Geometry check sheet. Reference: the model listing, model coordinates, mm. Face numbers are marked on the shaded views. A direction names the side the tool comes from. Coordinates: 2 decimals unless noted, no trailing zeros. Order: outer loops, then holes, each group sorted by start corner. A loop starts at its lowest first (then second) coordinate and runs counter-clockwise, first axis right, second up. Notation, with made-up numbers: (7.5, 83) - (22.5, 83) arc R25 cw to (22.5, 95) - close; hole circle Ø4 at (57.25, -14). An arc over 180 degrees is marked (long way). Use CSV: the item, a comma, the result in double quotes. Start each with the question number.
1) Thickness scan on probe 1 along X at (y, z) = (157, 1.2); probe 2 along Y at (x, z) = (15, 4.75); probe 3 along Y at (x, z) = (37.5, 3.3). Record the ranges inside material, lowest first. Write a range as [from, to].
2) Draft check along Y on the marked faces 3, 4 and 5. Enter one of: released by +Y, released by -Y, zero draft, split by the parting line, or undercut.
3) Tool access check on the marked faces 1 and 2. Record the directions out of +Z, -Z, +X, -X, +Y, -Y that give a thin tool (end or side, any length) a straight path to the whole face; none if there is none.
4) Depth check by flat-ended pin: P1, Ø3, axis at x = 2.5, y = 8.5, coming from the -Z side; P2, Ø2, axis at x = 27.5, z = 5.5, coming from the -Y side; P3, Ø0.8, axis at x = 37.5, z = 7.5, coming from the -Y side. Enter the tip coordinate at first touch or a pass-through.
5) Sectioned sample at A-A, the plane y = 55. Record the cut outline in (x, z).
from build123d import *

# Parameters (mm, degrees)
SKETCH_W        = 50
SKETCH_H        = 160
PAD_DEPTH       = 10
POCKET_DEPTH    = 7
SKETCH003_R     = 1.6
POCKET002_DEPTH = 10
POCKET003_DEPTH = 10
SKETCH005_W     = 6.1
SKETCH005_H     = 160
POCKET004_DEPTH = 3
POCKET005_DEPTH = 5.9
SKETCH007_W     = 160
SKETCH007_H     = 4.1
POCKET006_DEPTH = 5.9
SKETCH008_W     = 30
SKETCH008_H     = 140
POCKET007_DEPTH = 7
SKETCH009_W     = 5.7
SKETCH009_H     = 2.6
POCKET008_DEPTH = 6.15
SKETCH010_R     = 1.6
POCKET009_DEPTH = 10
SKETCH011_R     = 1.6
POCKET010_DEPTH = 10


with BuildPart() as part:
    # Sketch → Pad (new body)
    with BuildSketch(Plane.XY):
        with Locations((25, 80)):
            Rectangle(SKETCH_W, SKETCH_H)
    extrude(amount=PAD_DEPTH)

    # Sketch001 (on Face6 of Pad) → Pocket (cut)
    with BuildSketch(Plane.XY.offset(10)):
        Polygon((17.4, 6.1), (32.6, 6.1), (30.1, 0), (19.9, 0), align=None)
        Polygon((42.4, 6.1), (57.6, 6.1), (55.1, 0), (44.9, 0), align=None)
        Polygon((-7.6, 6.1), (7.6, 6.1), (5.1, 0), (-5.1, 0), align=None)
        Polygon((32.2, 153.9), (17.4, 153.9), (19.9, 160), (29.7, 160), align=None)
        Polygon((7.2, 153.9), (-7.6, 153.9), (-5.1, 160), (4.7, 160), align=None)
        Polygon((57.2, 153.9), (42.4, 153.9), (44.9, 160), (54.7, 160), align=None)
    extrude(amount=-POCKET_DEPTH, mode=Mode.SUBTRACT)

    # Sketch003 → Pocket002 (cut)
    with BuildSketch(Plane.XY.offset(10)):
        with Locations((12.5, 157)):
            Circle(SKETCH003_R)
        with Locations((37.5, 157)):
            Circle(SKETCH003_R)
        with Locations((12.5, 3)):
            Circle(SKETCH003_R)
        with Locations((37.5, 3)):
            Circle(SKETCH003_R)
    extrude(amount=-POCKET002_DEPTH, mode=Mode.SUBTRACT)

    # Sketch004 (on Face2 of Pocket002) → Pocket003 (cut)
    with BuildSketch(Plane(origin=(0, 0, 0), x_dir=(1, 0, 0), z_dir=(0, 0, -1))):
        Polygon((43.9, -84.9), (43.9, -100.1), (50, -97.6), (50, -87.4), align=None)
        Polygon((43.9, -59.9), (43.9, -75.1), (50, -72.6), (50, -62.4), align=None)
        Polygon((43.9, -34.9), (43.9, -50.1), (50, -47.6), (50, -37.4), align=None)
        Polygon((43.9, -9.9), (43.9, -25.1), (50, -22.6), (50, -12.4), align=None)
        Polygon((43.9, -134.9), (43.9, -150.1), (50, -147.6), (50, -137.4), align=None)
        Polygon((43.9, -109.9), (43.9, -125.1), (50, -122.6), (50, -112.4), align=None)
    extrude(amount=-POCKET003_DEPTH, mode=Mode.SUBTRACT)

    # Sketch005 (on Face2 of Pocket003) → Pocket004 (cut)
    with BuildSketch(Plane(origin=(0, 0, 0), x_dir=(1, 0, 0), z_dir=(0, 0, -1))):
        with Locations((46.95, -80)):
            Rectangle(SKETCH005_W, SKETCH005_H)
    extrude(amount=-POCKET004_DEPTH, mode=Mode.SUBTRACT)

    # Sketch006 (on Face12 of Pocket004) → Pocket005 (cut)
    with BuildSketch(Plane(origin=(0, 0, 0), x_dir=(0, -1, 0), z_dir=(-1, 0, 0))):
        Polygon((-100.1, 10), (-84.9, 10), (-87.4, 4.1), (-97.6, 4.1), align=None)
        Polygon((-75.1, 10), (-59.9, 10), (-62.4, 4.1), (-72.6, 4.1), align=None)
        Polygon((-150.1, 10), (-134.9, 10), (-137.4, 4.1), (-147.6, 4.1), align=None)
        Polygon((-125.1, 10), (-109.9, 10), (-112.4, 4.1), (-122.6, 4.1), align=None)
        Polygon((-50.1, 10), (-34.9, 10), (-37.4, 4.1), (-47.6, 4.1), align=None)
        Polygon((-25.1, 10), (-9.9, 10), (-12.4, 4.1), (-22.6, 4.1), align=None)
    extrude(amount=-POCKET005_DEPTH, mode=Mode.SUBTRACT)

    # Sketch007 (on Face12 of Pocket005) → Pocket006 (cut)
    with BuildSketch(Plane(origin=(0, 0, 0), x_dir=(0, -1, 0), z_dir=(-1, 0, 0))):
        with Locations((-80, 2.05)):
            Rectangle(SKETCH007_W, SKETCH007_H)
    extrude(amount=-POCKET006_DEPTH, mode=Mode.SUBTRACT)

    # Sketch008 (on Face2 of Pocket006) → Pocket007 (cut)
    with BuildSketch(Plane(origin=(0, 0, 0), x_dir=(1, 0, 0), z_dir=(0, 0, -1))):
        with Locations((25, -80)):
            Rectangle(SKETCH008_W, SKETCH008_H)
    extrude(amount=-POCKET007_DEPTH, mode=Mode.SUBTRACT)

    # Sketch009 (on Face6 of Pocket007) → Pocket008 (cut)
    with BuildSketch(Plane.XY.offset(10)):
        with Locations((12.5, 157)):
            Rectangle(SKETCH009_W, SKETCH009_H)
        with Locations((37.5, 157)):
            Rectangle(SKETCH009_W, SKETCH009_H)
        with Locations((12.5, 3)):
            Rectangle(SKETCH009_W, SKETCH009_H)
        with Locations((37.5, 3)):
            Rectangle(SKETCH009_W, SKETCH009_H)
    extrude(amount=-POCKET008_DEPTH, mode=Mode.SUBTRACT)

    # Sketch010 (on Face15 of Pocket008) → Pocket009 (cut)
    with BuildSketch(Plane.XZ):
        with Locations((12.5, 7)):
            Circle(SKETCH010_R)
        with Locations((37.5, 7)):
            Circle(SKETCH010_R)
    extrude(amount=-POCKET009_DEPTH, mode=Mode.SUBTRACT)

    # Sketch011 (on Face1 of Pocket009) → Pocket010 (cut)
    with BuildSketch(Plane(origin=(0, 160, 0), x_dir=(-1, 0, 0), z_dir=(0, 1, 0))):
        with Locations((-37.5, 7)):
            Circle(SKETCH011_R)
        with Locations((-12.5, 7)):
            Circle(SKETCH011_R)
    extrude(amount=-POCKET010_DEPTH, mode=Mode.SUBTRACT)


solid = part.part
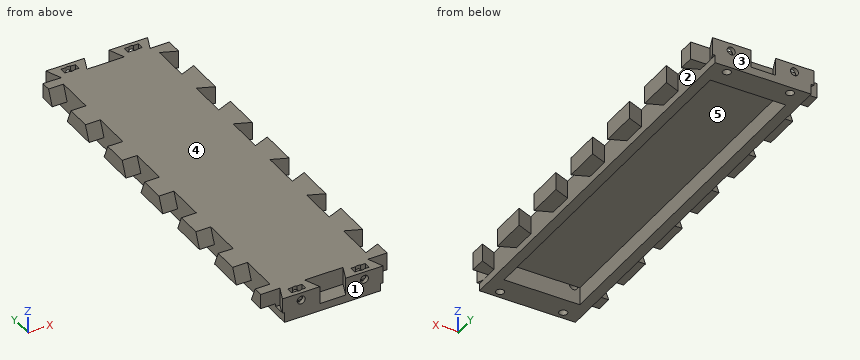
Evaluation:
1,probe 1,"[5.9, 10.9], [14.1, 35.9], [39.1, 43.9]"
1,probe 2,"[0, 1.7], [4.3, 10], [150, 155.7], [158.3, 160]"
1,probe 3,"[0, 1.4], [4.6, 10], [150, 155.4], [158.6, 160]"
2,face 3,"released by +Y"
2,face 4,"zero draft"
2,face 5,"undercut"
3,face 1,"+Z, -Z, +X, -X, -Y"
3,face 2,"-Z"
4,P1,"z = 4.1"
4,P2,"y = 6.1"
4,P3,"y = 10"
5,outline,"(0, 4.1) - (5.9, 4.1) - (5.9, 0) - (10, 0) - (10, 7) - (40, 7) - (40, 0) - (43.9, 0) - (43.9, 3) - (50, 3) - (50, 10) - (0, 10) - close"
